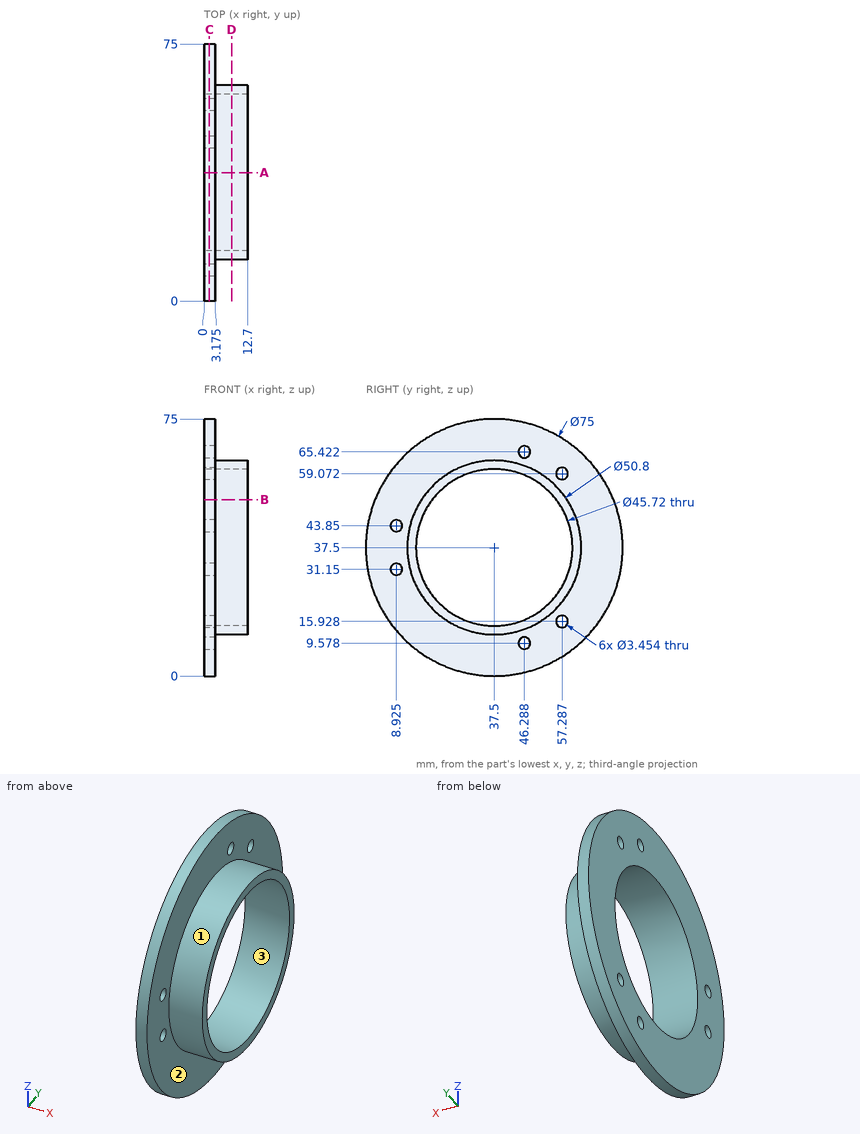
Job drawing, mm, ordinate dimensions from the low corner. One solid piece. Give positions to 0.01 mm unless a question says otherwise; leave off trailing zeros. Loops run counter-clockwise (first coordinate to the right, second up) from the corner with the lowest first, then second, coordinate; pieces in that order, holes last. Notation, with made-up numbers: M 8,89 L 46,89 A33 ccw 46,126 Z; hole C -30,-17.75 d6. An arc over 180 degrees is marked long. Answer in a Markdown table with one row per item. Add a question column.
Item 1: Probe probe 1 along Y at (x, z) = (11, 38) (1 decimal); probe 2 along X at (y, z) = (71.5, 38) (1 decimal); probe 3 along Z at (x, y) = (1.5, 58) (1 decimal). List the from-to ranges inside material, lowest first.
Item 2: Band-saw the part on A-A on y = 37.5. Give the cut face in (x, z) (1 decimal).
Item 3: Drop flat-ended pins along their axis: P1, Ø3, axis at x = 4, z = 9, coming from the -Y side (1 decimal); P2, Ø3, axis at x = 1.5, y = 54.5, coming from the +Z side; P3, Ø2, axis at x = 5, z = 53.5, coming from the -Y side. Give the stop position or say it passes through.
Item 4: Band-saw the part on D-D on x = 8. Give the cut face in (y, z), then the cut area to 3 significant figures.
Item 5: Mould opens along Z. For the marked faces 1, 2 and 3 say: +Z half, -Z half, draft (parallel to the pull), parting line (faces both ways), or undercut.
Item 6: Band-saw the part on B-B on z = 51.5. Give the cut face in (x, y) (1 decimal), then the cut area to 3 significant figures.
Item 7: Band-saw the part on C-C on x = 1.5. Give the number of separate pieces and of enclosed holes in the cut face, then the cut area to 3 significant figures.
Reply:
| question | item | result |
|---|---|---|
| 1 | probe 1 | y = 12.1 to 14.6, 60.4 to 62.9 |
| 1 | probe 2 | x = 0 to 3.2 |
| 1 | probe 3 | z = 6.1 to 14.4, 17.5 to 27.4, 47.6 to 57.5, 60.6 to 68.9 |
| 2 | outline | M 0,0 L 3.2,0 L 3.2,12.1 L 12.7,12.1 L 12.7,14.6 L 0,14.6 Z; M 0,60.4 L 12.7,60.4 L 12.7,62.9 L 3.2,62.9 L 3.2,75 L 0,75 Z |
| 3 | P1 | stops at y = 11.7 |
| 3 | P2 | stops at z = 71.65 |
| 3 | P3 | stops at y = 17 |
| 4 | outline | C 37.5,37.5 d50.8; hole C 37.5,37.5 d45.72 |
| 4 | area | 385 mm^2 |
| 5 | face 1 | parting line |
| 5 | face 2 | draft |
| 5 | face 3 | undercut |
| 6 | outline | M 0,2.7 L 3.2,2.7 L 3.2,16.3 L 12.7,16.3 L 12.7,19.4 L 0,19.4 Z; M 0,55.6 L 12.7,55.6 L 12.7,58.7 L 3.2,58.7 L 3.2,72.3 L 0,72.3 Z |
| 6 | area | 166 mm^2 |
| 7 | separate pieces | 1 |
| 7 | enclosed holes | 7 |
| 7 | area | 2,720 mm^2 |
